Can you work these out from the model? Positions are in its coordinate system, mm. A direction names the side the tool comes from. Coordinates: 2 decimals unless noted, no trailing zeros. Loops run counter-clockwise (first coordinate to the right, second up) from the corner with the lowest first, then second, coordinate; pieces in that order, holes last. Notation, with made-up numbers: M -37.5,70 L 16.5,70 A19 cw 16.5,105 Z; hole C -24,-24.5 d4. An arc over 180 degrees is marked long. Return JSON: item names as keys, results as strings. Group by question number.
```python
from build123d import *

# Parameters (mm, degrees)
SKETCH1_W           = 1800
SKETCH1_H           = 650
BOSS_EXTRUDE1_DEPTH = 30
SKETCH2_W           = 50
SKETCH2_H           = 30
BOSS_EXTRUDE2_DEPTH = 540
SKETCH3_W           = 1800
SKETCH3_H           = 30
BOSS_EXTRUDE4_DEPTH = 150
SKETCH4_W           = 30
SKETCH4_H           = 150
BOSS_EXTRUDE5_DEPTH = 620
SKETCH5_W           = 100
SKETCH5_H           = 30
BOSS_EXTRUDE6_DEPTH = 240
SKETCH6_W           = 50
SKETCH6_H           = 30
BOSS_EXTRUDE7_DEPTH = 100
SKETCH7_W           = 50
SKETCH7_H           = 40
BOSS_EXTRUDE8_DEPTH = 140
SKETCH8_W           = 50
SKETCH8_H           = 10
CUT_EXTRUDE1_DEPTH  = 20
SKETCH9_R           = 25
CUT_EXTRUDE2_DEPTH  = 40
SKETCH10_R          = 25
CUT_EXTRUDE3_DEPTH  = 40
SKETCH11_R          = 25
CUT_EXTRUDE4_DEPTH  = 40


with BuildPart() as part:
    # Sketch1 → Boss-Extrude1 (new body)
    with BuildSketch(Plane.XY):
        Rectangle(SKETCH1_W, SKETCH1_H)
    extrude(amount=-BOSS_EXTRUDE1_DEPTH)

    # Sketch2 → Boss-Extrude2 (add)
    with BuildSketch(Plane.XY):
        with Locations((75, -310)):
            Rectangle(SKETCH2_W, SKETCH2_H)
        with Locations((-815, -310)):
            Rectangle(SKETCH2_W, SKETCH2_H)
    extrude(amount=BOSS_EXTRUDE2_DEPTH)

    # Sketch3 → Boss-Extrude4 (add)
    with BuildSketch(Plane.XY.offset(540)):
        with Locations((0, -310)):
            Rectangle(SKETCH3_W, SKETCH3_H)
    extrude(amount=BOSS_EXTRUDE4_DEPTH)

    # Sketch4 → Boss-Extrude5 (add)
    with BuildSketch(Plane(origin=(0, -295, 0), x_dir=(1, 0, 0), z_dir=(0, 1, 0))):
        with Locations((65, -345)):
            Rectangle(SKETCH4_W, SKETCH4_H)
    extrude(amount=BOSS_EXTRUDE5_DEPTH)

    # Sketch5 → Boss-Extrude6 (add)
    with BuildSketch(Plane.XY.offset(690)):
        with Locations((-730, -310)):
            Rectangle(SKETCH5_W, SKETCH5_H)
    extrude(amount=BOSS_EXTRUDE6_DEPTH)

    # Sketch6 → Boss-Extrude7 (add)
    with BuildSketch(Plane.XY.offset(690)):
        with Locations((-455, -310)):
            Rectangle(SKETCH6_W, SKETCH6_H)
    extrude(amount=BOSS_EXTRUDE7_DEPTH)

    # Sketch7 → Boss-Extrude8 (add)
    with BuildSketch(Plane(origin=(0, -295, 0), x_dir=(1, 0, 0), z_dir=(0, 1, 0))):
        with Locations((-455, -770)):
            Rectangle(SKETCH7_W, SKETCH7_H)
    extrude(amount=BOSS_EXTRUDE8_DEPTH)

    # Sketch8 → Cut-Extrude1 (cut)
    with BuildSketch(Plane(origin=(0, -155, 0), x_dir=(1, 0, 0), z_dir=(0, 1, 0))):
        with Locations((-455, -775)):
            Rectangle(SKETCH8_W, SKETCH8_H)
    extrude(amount=-CUT_EXTRUDE1_DEPTH, mode=Mode.SUBTRACT)

    # Sketch9 → Cut-Extrude2 (cut)
    with BuildSketch(Plane.XZ.offset(325)):
        with Locations(Location((750, 615, 0), (0, 0, 270))):
            Circle(SKETCH9_R)
        with Locations(Location((530, 615, 0), (0, 0, 270))):
            Circle(SKETCH9_R)
        with Locations(Location((310, 615, 0), (0, 0, 270))):
            Circle(SKETCH9_R)
    extrude(amount=-CUT_EXTRUDE2_DEPTH, mode=Mode.SUBTRACT)

    # Sketch10 → Cut-Extrude3 (cut)
    with BuildSketch(Plane.ZY.offset(-50)):
        with Locations((345, -95)):
            Circle(SKETCH10_R)
        with Locations((345, 175)):
            Circle(SKETCH10_R)
    extrude(amount=-CUT_EXTRUDE3_DEPTH, mode=Mode.SUBTRACT)

    # Sketch11 → Cut-Extrude4 (cut)
    with BuildSketch(Plane.XZ.offset(325)):
        with Locations(Location((-730, 810, 0), (0, 0, 270))):
            Circle(SKETCH11_R)
    extrude(amount=-CUT_EXTRUDE4_DEPTH, mode=Mode.SUBTRACT)


solid = part.part
```
1) For pin 1 (15 mm diameter, centred on x = 466.5, y = -307, fed in from +Z); pin 2 (24 mm diameter, centred on x = 64.5, y = 141, fed in from +Z); pin 3 (3 mm diameter, centred on x = 319.5, y = -127, fed in from +Z), each with a flat end and sliding along its axis, tell me the tip position at first contact or that it passes through.
2) Suppose I cut it at D-D, the plane z = 345. List the corners of the cut face in (x, y) for me.
3) Suppose I cut it at B-B, the plane y = -44. List the corners of the cut face in (x, z) for me.
4) If we mould it in two halves opening along Z, with no side actions, what happens to faces 1 (the face through (-752.2, -310.2, 798.5)), 2 (the face through (-13, 5, -30)), 3 (the face through (-138, -325, 554))? For each: +Z half, -Z half, draft (parallel to the pull), parting line (faces both ways), or undercut.
5) Suppose I cut it at A-A, the plane z = 810. List the corners of the cut face in (x, y) for me, then the cut area to 3 significant figures.
6) For faces 4 (the face through (80, 11, 346)), 5 (the face through (-455, -226, 750)), 6 (the face through (-480, -260, 752)), which set-ups out of +Z, -Z, +X, -X, +Y, -Y let a thin tool reach every point of the face, with its end or its side?
7) Suppose I cut it at C-C, the plane x = 310. List the corners of the cut face in (y, z) for me, then the cut area to 3 significant figures.
8) If I drill on line 1 (Y direction, x = 69.25, z = 345); line 2 (X direction, y = -312, z = 615); line 3 (Z direction, x = 335, y = -54), over which ranges is the centre line in solid material (lowest first)? Write a range as from..to.
Returned:
{
 "1": {"pin 1": "stops at z = 690", "pin 2": "stops at z = 420", "pin 3": "stops at z = 0"},
 "2": {"outline": "M -840,-325 L -790,-325 L -790,-295 L -840,-295 Z; M 50,-325 L 100,-325 L 100,-295 L 80,-295 L 80,-120 L 50,-120 Z; M 50,-70 L 80,-70 L 80,150 L 50,150 Z; M 50,200 L 80,200 L 80,325 L 50,325 Z"},
 "3": {"outline": "M -900,-30 L 900,-30 L 900,0 L -900,0 Z; M 50,270 L 80,270 L 80,420 L 50,420 Z"},
 "4": {"face 1": "undercut", "face 2": "-Z half", "face 3": "draft"},
 "5": {"outline": "M -780,-325 L -755,-325 L -755,-295 L -780,-295 Z; M -705,-325 L -680,-325 L -680,-295 L -705,-295 Z", "area": "1,500 mm²"},
 "6": {"face 4": "+Z, +X, +Y", "face 5": "+X, -X, +Y", "face 6": "+Z, +Y, -Y"},
 "7": {"outline": "M -325,-30 L 325,-30 L 325,0 L -325,0 Z; M -325,540 L -295,540 L -295,590 L -325,590 Z; M -325,640 L -295,640 L -295,690 L -325,690 Z", "area": "22,500 mm²"},
 "8": {"line 1": "y = -325..-120, -70..150, 200..325", "line 2": "x = -900..285, 335..505, 555..725, 775..900", "line 3": "z = -30..0"}
}
